from build123d import *

# Parameters (mm, degrees)
BOSS_EXTRUDE1_DEPTH = 4
CAVITY1_START       = 3
CAVITY1_OUTLINE_R   = 0.5
CAVITY1_OUTLINE_R_2 = 0.384
CAVITY1_DEPTH       = 1
CAVITY1_2_DEPTH     = 3
CAVITY1_START_2     = 1
CAVITY1_3_OUTLINE_R = 0.384
CAVITY1_3_DEPTH     = 2


# Read off the part's stored shape, not the designer's step: Cavity1
with BuildPart() as part:
    # Sketch1 → Boss-Extrude1 (new body)
    with BuildSketch(Plane(origin=(0, 0, 0), x_dir=(1, 0, 0), z_dir=(0, 1, 0))):
        Polygon((6.92820323, 0), (3.464101615, 6), (-3.464101615, 6), (-6.92820323, 0), (-3.464101615, -6), (3.464101615, -6), align=None)
    extrude(amount=BOSS_EXTRUDE1_DEPTH)

    # Cavity1 outline → Cavity1 (cut)
    # profile 1 of 20: a face of its own
    with BuildSketch(Plane(origin=(0, 0, 0), x_dir=(1, 0, 0), z_dir=(0, 1, 0)).offset(CAVITY1_START)):
        Polygon((3.464101615, -6), (6.92820323, 0), (3.464101615, 6), (-3.464101615, 6), (-6.92820323, 0), (-3.464101615, -6), align=None)
        with Locations((-2.053589838, -4.156921938)):
            Circle(CAVITY1_OUTLINE_R, mode=Mode.SUBTRACT)
        with Locations((-4.453589838, 0)):
            Circle(CAVITY1_OUTLINE_R, mode=Mode.SUBTRACT)
        with Locations((-3.253589838, -2.078460969)):
            Circle(CAVITY1_OUTLINE_R, mode=Mode.SUBTRACT)
        with Locations((-0.853589838, -2.078460969)):
            Circle(CAVITY1_OUTLINE_R, mode=Mode.SUBTRACT)
        with Locations((-2.053589838, 0)):
            Circle(CAVITY1_OUTLINE_R, mode=Mode.SUBTRACT)
        with Locations((0.346410162, -4.156921938)):
            Circle(CAVITY1_OUTLINE_R, mode=Mode.SUBTRACT)
        with Locations((2.746410162, -4.156921938)):
            Circle(CAVITY1_OUTLINE_R, mode=Mode.SUBTRACT)
        with Locations((1.546410162, -2.078460969)):
            Circle(CAVITY1_OUTLINE_R, mode=Mode.SUBTRACT)
        with Locations((0.346410162, 0)):
            Circle(CAVITY1_OUTLINE_R, mode=Mode.SUBTRACT)
        with Locations((2.746410162, 0)):
            Circle(CAVITY1_OUTLINE_R, mode=Mode.SUBTRACT)
        with Locations((3.946410162, -2.078460969)):
            Circle(CAVITY1_OUTLINE_R, mode=Mode.SUBTRACT)
        with Locations((5.146410162, 0)):
            Circle(CAVITY1_OUTLINE_R, mode=Mode.SUBTRACT)
        with Locations((-3.253589838, 2.078460969)):
            Circle(CAVITY1_OUTLINE_R, mode=Mode.SUBTRACT)
        with Locations((-0.853589838, 2.078460969)):
            Circle(CAVITY1_OUTLINE_R, mode=Mode.SUBTRACT)
        with Locations((-2.053589838, 4.156921938)):
            Circle(CAVITY1_OUTLINE_R, mode=Mode.SUBTRACT)
        with Locations((1.546410162, 2.078460969)):
            Circle(CAVITY1_OUTLINE_R, mode=Mode.SUBTRACT)
        with Locations((3.946410162, 2.078460969)):
            Circle(CAVITY1_OUTLINE_R, mode=Mode.SUBTRACT)
        with Locations((0.346410162, 4.156921938)):
            Circle(CAVITY1_OUTLINE_R, mode=Mode.SUBTRACT)
        with Locations((2.746410162, 4.156921938)):
            Circle(CAVITY1_OUTLINE_R, mode=Mode.SUBTRACT)
    # profile 2 of 20: a face of its own
    with BuildSketch(Plane(origin=(0, 0, 0), x_dir=(1, 0, 0), z_dir=(0, 1, 0)).offset(CAVITY1_START)):
        with Locations((0.346410162, 0)):
            Circle(CAVITY1_OUTLINE_R_2)
    # profile 3 of 20: a face of its own
    with BuildSketch(Plane(origin=(0, 0, 0), x_dir=(1, 0, 0), z_dir=(0, 1, 0)).offset(CAVITY1_START)):
        with Locations((3.946410162, 2.078460969)):
            Circle(CAVITY1_OUTLINE_R_2)
    # profile 4 of 20: a face of its own
    with BuildSketch(Plane(origin=(0, 0, 0), x_dir=(1, 0, 0), z_dir=(0, 1, 0)).offset(CAVITY1_START)):
        with Locations((5.146410162, 0)):
            Circle(CAVITY1_OUTLINE_R_2)
    # profile 5 of 20: a face of its own
    with BuildSketch(Plane(origin=(0, 0, 0), x_dir=(1, 0, 0), z_dir=(0, 1, 0)).offset(CAVITY1_START)):
        with Locations((2.746410162, 0)):
            Circle(CAVITY1_OUTLINE_R_2)
    # profile 6 of 20: a face of its own
    with BuildSketch(Plane(origin=(0, 0, 0), x_dir=(1, 0, 0), z_dir=(0, 1, 0)).offset(CAVITY1_START)):
        with Locations((0.346410162, 4.156921938)):
            Circle(CAVITY1_OUTLINE_R_2)
    # profile 7 of 20: a face of its own
    with BuildSketch(Plane(origin=(0, 0, 0), x_dir=(1, 0, 0), z_dir=(0, 1, 0)).offset(CAVITY1_START)):
        with Locations((2.746410162, 4.156921938)):
            Circle(CAVITY1_OUTLINE_R_2)
    # profile 8 of 20: a face of its own
    with BuildSketch(Plane(origin=(0, 0, 0), x_dir=(1, 0, 0), z_dir=(0, 1, 0)).offset(CAVITY1_START)):
        with Locations((1.546410162, 2.078460969)):
            Circle(CAVITY1_OUTLINE_R_2)
    # profile 9 of 20: a face of its own
    with BuildSketch(Plane(origin=(0, 0, 0), x_dir=(1, 0, 0), z_dir=(0, 1, 0)).offset(CAVITY1_START)):
        with Locations((-3.253589838, 2.078460969)):
            Circle(CAVITY1_OUTLINE_R_2)
    # profile 10 of 20: a face of its own
    with BuildSketch(Plane(origin=(0, 0, 0), x_dir=(1, 0, 0), z_dir=(0, 1, 0)).offset(CAVITY1_START)):
        with Locations((-2.053589838, 4.156921938)):
            Circle(CAVITY1_OUTLINE_R_2)
    # profile 11 of 20: a face of its own
    with BuildSketch(Plane(origin=(0, 0, 0), x_dir=(1, 0, 0), z_dir=(0, 1, 0)).offset(CAVITY1_START)):
        with Locations((-0.853589838, 2.078460969)):
            Circle(CAVITY1_OUTLINE_R_2)
    # profile 12 of 20: a face of its own
    with BuildSketch(Plane(origin=(0, 0, 0), x_dir=(1, 0, 0), z_dir=(0, 1, 0)).offset(CAVITY1_START)):
        with Locations((-3.253589838, -2.078460969)):
            Circle(CAVITY1_OUTLINE_R_2)
    # profile 13 of 20: a face of its own
    with BuildSketch(Plane(origin=(0, 0, 0), x_dir=(1, 0, 0), z_dir=(0, 1, 0)).offset(CAVITY1_START)):
        with Locations((-4.453589838, 0)):
            Circle(CAVITY1_OUTLINE_R_2)
    # profile 14 of 20: a face of its own
    with BuildSketch(Plane(origin=(0, 0, 0), x_dir=(1, 0, 0), z_dir=(0, 1, 0)).offset(CAVITY1_START)):
        with Locations((-2.053589838, 0)):
            Circle(CAVITY1_OUTLINE_R_2)
    # profile 15 of 20: a face of its own
    with BuildSketch(Plane(origin=(0, 0, 0), x_dir=(1, 0, 0), z_dir=(0, 1, 0)).offset(CAVITY1_START)):
        with Locations((0.346410162, -4.156921938)):
            Circle(CAVITY1_OUTLINE_R_2)
    # profile 16 of 20: a face of its own
    with BuildSketch(Plane(origin=(0, 0, 0), x_dir=(1, 0, 0), z_dir=(0, 1, 0)).offset(CAVITY1_START)):
        with Locations((-2.053589838, -4.156921938)):
            Circle(CAVITY1_OUTLINE_R_2)
    # profile 17 of 20: a face of its own
    with BuildSketch(Plane(origin=(0, 0, 0), x_dir=(1, 0, 0), z_dir=(0, 1, 0)).offset(CAVITY1_START)):
        with Locations((-0.853589838, -2.078460969)):
            Circle(CAVITY1_OUTLINE_R_2)
    # profile 18 of 20: a face of its own
    with BuildSketch(Plane(origin=(0, 0, 0), x_dir=(1, 0, 0), z_dir=(0, 1, 0)).offset(CAVITY1_START)):
        with Locations((3.946410162, -2.078460969)):
            Circle(CAVITY1_OUTLINE_R_2)
    # profile 19 of 20: a face of its own
    with BuildSketch(Plane(origin=(0, 0, 0), x_dir=(1, 0, 0), z_dir=(0, 1, 0)).offset(CAVITY1_START)):
        with Locations((2.746410162, -4.156921938)):
            Circle(CAVITY1_OUTLINE_R_2)
    # profile 20 of 20: a face of its own
    with BuildSketch(Plane(origin=(0, 0, 0), x_dir=(1, 0, 0), z_dir=(0, 1, 0)).offset(CAVITY1_START)):
        with Locations((1.546410162, -2.078460969)):
            Circle(CAVITY1_OUTLINE_R_2)
    extrude(amount=CAVITY1_DEPTH, mode=Mode.SUBTRACT)

    # Cavity1 2 outline → Cavity1 2 (cut)
    with BuildSketch(Plane(origin=(0, 0, 0), x_dir=(1, 0, 0), z_dir=(0, 1, 0))):
        Polygon((3.464101615, -6), (6.92820323, 0), (3.464101615, 6), (-3.464101615, 6), (-6.92820323, 0), (-3.464101615, -6), align=None)
        Polygon((6.466323015, 0), (3.406366588, -5.3), (-2.713546265, -5.3), (-5.773502692, 0), (-2.713546265, 5.3), (3.406366588, 5.3), align=None, mode=Mode.SUBTRACT)
    extrude(amount=CAVITY1_2_DEPTH, mode=Mode.SUBTRACT)

    # Cavity1 3 outline → Cavity1 3 (cut)
    with BuildSketch(Plane(origin=(0, 0, 0), x_dir=(1, 0, 0), z_dir=(0, 1, 0)).offset(CAVITY1_START_2)):
        with Locations((0.346410162, 0)):
            Circle(CAVITY1_3_OUTLINE_R)
        with Locations((3.946410162, 2.078460969)):
            Circle(CAVITY1_3_OUTLINE_R)
        with Locations((5.146410162, 0)):
            Circle(CAVITY1_3_OUTLINE_R)
        with Locations((2.746410162, 0)):
            Circle(CAVITY1_3_OUTLINE_R)
        with Locations((0.346410162, 4.156921938)):
            Circle(CAVITY1_3_OUTLINE_R)
        with Locations((2.746410162, 4.156921938)):
            Circle(CAVITY1_3_OUTLINE_R)
        with Locations((1.546410162, 2.078460969)):
            Circle(CAVITY1_3_OUTLINE_R)
        with Locations((-3.253589838, 2.078460969)):
            Circle(CAVITY1_3_OUTLINE_R)
        with Locations((-2.053589838, 4.156921938)):
            Circle(CAVITY1_3_OUTLINE_R)
        with Locations((-0.853589838, 2.078460969)):
            Circle(CAVITY1_3_OUTLINE_R)
        with Locations((-3.253589838, -2.078460969)):
            Circle(CAVITY1_3_OUTLINE_R)
        with Locations((-4.453589838, 0)):
            Circle(CAVITY1_3_OUTLINE_R)
        with Locations((-2.053589838, 0)):
            Circle(CAVITY1_3_OUTLINE_R)
        with Locations((0.346410162, -4.156921938)):
            Circle(CAVITY1_3_OUTLINE_R)
        with Locations((-2.053589838, -4.156921938)):
            Circle(CAVITY1_3_OUTLINE_R)
        with Locations((-0.853589838, -2.078460969)):
            Circle(CAVITY1_3_OUTLINE_R)
        with Locations((3.946410162, -2.078460969)):
            Circle(CAVITY1_3_OUTLINE_R)
        with Locations((2.746410162, -4.156921938)):
            Circle(CAVITY1_3_OUTLINE_R)
        with Locations((1.546410162, -2.078460969)):
            Circle(CAVITY1_3_OUTLINE_R)
    extrude(amount=CAVITY1_3_DEPTH, mode=Mode.SUBTRACT)


solid = part.part
Input: part model. Units: mm. Frame: model coordinates. Round coordinates to 2 decimals unless told otherwise and drop trailing zeros. Order: outer loops, then holes, each group sorted by start corner. A loop starts at its lowest first (then second) coordinate and runs counter-clockwise, first axis right, second up. Notation, with made-up numbers: (-34.5, 57.5) - (-15.5, 57.5) arc R24 cw to (-15.5, 73.5) - close; hole circle Ø4 at (-22.75, 42.25). An arc over 180 degrees is marked (long way). Answer as a JSON object with one key per item and string values. Group by question number.
(1) Cut plane B-B (x = -3.5). Return loops of the section in (y, z), then the cut area to 3 significant figures.
(2) Cut plane D-D (y = 0.65). Return loops of the section in (x, z), then the cut area to 3 significant figures.
(3) Cut plane C-C (z = -4). Return loops of the section in (x, y).
(4) Cut plane A-A (y = 3.25). Count the separate pieces of the cut face and the enclosed holes in it, then the cut area to 3 significant figures.
(5) Pin query (flat end, axial travel): P1, Ø1.5, axis at y = 2, z = -3.5, coming from the +X side; P2, Ø0.6, axis at x = -2, z = 0, coming from the +Y side. Return the tip coordinate at first contact, or that it passes through.
(6) Draft query along Z for faces 1 (the face through (0, 3, -1)), 2 (the face through (0, 0, 0)), 3 (the face through (-4.22, 1.48, 2.69)). Return one class per face: released by +Z, released by -Z, zero draft, split by the parting line, or undercut.
(7) Material intervals for probe 1 along Z at (x, y) = (2.75, 2.6); probe 2 along Z at (x, y) = (1.25, 1.9); probe 3 along Y at (x, z) = (-2, -4.25), sorted ascending. Write a range as from..to.
Here are the results:
{
 "1": {"outline": "(0, -3.94) - (3, -3.94) - (3, -2.51) - (4, -2.51) - (4, -2.37) - (1, -2.37) - (1, -1.78) - (4, -1.78) - (4, -1.64) - (3, -1.64) - (3, 1.64) - (4, 1.64) - (4, 1.78) - (1, 1.78) - (1, 2.37) - (4, 2.37) - (4, 2.51) - (3, 2.51) - (3, 3.94) - (0, 3.94) - close", "area": "21.8 mm^2"},
 "2": {"outline": "(-5.77, 0) - (-2.71, -5.3) - (3.41, -5.3) - (6.47, 0) - (3.41, 5.3) - (-2.71, 5.3) - close", "area": "97.3 mm^2"},
 "3": {"outline": "(-3.46, 0) - (4.16, 0) - (4.16, 3) - (3.22, 3) - (3.22, 4) - (3.1, 4) - (3.1, 1) - (2.4, 1) - (2.4, 4) - (2.27, 4) - (2.27, 3) - (0.82, 3) - (0.82, 4) - (0.7, 4) - (0.7, 1) - (0, 1) - (0, 4) - (-0.13, 4) - (-0.13, 3) - (-1.58, 3) - (-1.58, 4) - (-1.7, 4) - (-1.7, 1) - (-2.4, 1) - (-2.4, 4) - (-2.53, 4) - (-2.53, 3) - (-3.46, 3) - close"},
 "4": {"separate pieces": "19", "enclosed holes": "19", "area": "6.12 mm^2"},
 "5": {"P1": "stops at x = 4.88", "P2": "stops at y = 1"},
 "6": {"face 1": "undercut", "face 2": "zero draft", "face 3": "released by +Z"},
 "7": {"probe 1": "z = -5.3..-4.54, -3.77..-0.38, 0.38..3.77, 4.54..5.3", "probe 2": "z = -5.3..-2.32, -1.83..1.83, 2.32..5.3", "probe 3": "y = 0..1"}
}
